```python
from build123d import *

# Parameters (mm, degrees)
F0_R          = 3
F0_R_2        = 2.5
F1_DEPTH      = 300
F2_R          = 2
F3_R          = 7
F5_DEPTH      = 30
F5_DEPTH_BACK = 30


# Not quite as in the source:
# - a feature names something its author has since deleted; it is built from what else it names


with BuildPart() as f1:
    # F0 (on Top) → F1 (new body)
    with BuildSketch(Plane.XY):
        with BuildLine():
            Line((18.15, -30), (30, -30))
            Line((30, -30), (30, -18.15))
            Line((30, -18.15), (27.5, -18.15))
            Line((27.5, -18.15), (27.5, -20.15))
            Line((27.5, -20.15), (21.5477069044, -20.15))
            ThreePointArc((21.5477069044, -20.15), (19.5, -15), (21.5477069044, -9.85))
            Line((21.5477069044, -9.85), (27.5, -9.85))
            Line((27.5, -9.85), (27.5, -11.85))
            Line((27.5, -11.85), (30, -11.85))
            Line((30, -11.85), (30, 11.85))
            Line((30, 11.85), (27.5, 11.85))
            Line((27.5, 11.85), (27.5, 9.85))
            Line((27.5, 9.85), (21.5477069044, 9.85))
            ThreePointArc((21.5477069044, 9.85), (19.5, 15), (21.5477069044, 20.15))
            Line((21.5477069044, 20.15), (27.5, 20.15))
            Line((27.5, 20.15), (27.5, 18.15))
            Line((27.5, 18.15), (30, 18.15))
            Line((30, 18.15), (30, 30))
            Line((30, 30), (18.15, 30))
            Line((18.15, 30), (18.15, 27.5))
            Line((18.15, 27.5), (20.15, 27.5))
            Line((20.15, 27.5), (20.15, 21.5477069044))
            ThreePointArc((20.15, 21.5477069044), (15, 19.5), (9.85, 21.5477069044))
            Line((9.85, 21.5477069044), (9.85, 27.5))
            Line((9.85, 27.5), (11.85, 27.5))
            Line((11.85, 27.5), (11.85, 30))
            Line((11.85, 30), (-11.85, 30))
            Line((-11.85, 30), (-11.85, 27.5))
            Line((-11.85, 27.5), (-9.85, 27.5))
            Line((-9.85, 27.5), (-9.85, 21.5477069044))
            ThreePointArc((-9.85, 21.5477069044), (-15, 19.5), (-20.15, 21.5477069044))
            Line((-20.15, 21.5477069044), (-20.15, 27.5))
            Line((-20.15, 27.5), (-18.15, 27.5))
            Line((-18.15, 27.5), (-18.15, 30))
            Line((-18.15, 30), (-30, 30))
            Line((-30, 30), (-30, 18.15))
            Line((-30, 18.15), (-27.5, 18.15))
            Line((-27.5, 18.15), (-27.5, 20.15))
            Line((-27.5, 20.15), (-21.5477069044, 20.15))
            ThreePointArc((-21.5477069044, 20.15), (-19.5, 15), (-21.5477069044, 9.85))
            Line((-21.5477069044, 9.85), (-27.5, 9.85))
            Line((-27.5, 9.85), (-27.5, 11.85))
            Line((-27.5, 11.85), (-30, 11.85))
            Line((-30, 11.85), (-30, -11.85))
            Line((-30, -11.85), (-27.5, -11.85))
            Line((-27.5, -11.85), (-27.5, -9.85))
            Line((-27.5, -9.85), (-21.5477069044, -9.85))
            ThreePointArc((-21.5477069044, -9.85), (-19.5, -15), (-21.5477069044, -20.15))
            Line((-21.5477069044, -20.15), (-27.5, -20.15))
            Line((-27.5, -20.15), (-27.5, -18.15))
            Line((-27.5, -18.15), (-30, -18.15))
            Line((-30, -18.15), (-30, -30))
            Line((-30, -30), (-18.15, -30))
            Line((-18.15, -30), (-18.15, -27.5))
            Line((-18.15, -27.5), (-20.15, -27.5))
            Line((-20.15, -27.5), (-20.15, -21.5477069044))
            ThreePointArc((-20.15, -21.5477069044), (-15, -19.5), (-9.85, -21.5477069044))
            Line((-9.85, -21.5477069044), (-9.85, -27.5))
            Line((-9.85, -27.5), (-11.85, -27.5))
            Line((-11.85, -27.5), (-11.85, -30))
            Line((-11.85, -30), (11.85, -30))
            Line((11.85, -30), (11.85, -27.5))
            Line((11.85, -27.5), (9.85, -27.5))
            Line((9.85, -27.5), (9.85, -21.5477069044))
            ThreePointArc((9.85, -21.5477069044), (15, -19.5), (20.15, -21.5477069044))
            Line((20.15, -21.5477069044), (20.15, -27.5))
            Line((20.15, -27.5), (18.15, -27.5))
            Line((18.15, -27.5), (18.15, -30))
        make_face()
        with Locations((-25, -25)):
            Circle(F0_R, mode=Mode.SUBTRACT)
        with Locations((-15, -15)):
            Circle(F0_R_2, mode=Mode.SUBTRACT)
        with Locations((25, -25)):
            Circle(F0_R, mode=Mode.SUBTRACT)
        with Locations((15, -15)):
            Circle(F0_R_2, mode=Mode.SUBTRACT)
        with Locations((-25, 25)):
            Circle(F0_R, mode=Mode.SUBTRACT)
        with Locations((-15, 15)):
            Circle(F0_R_2, mode=Mode.SUBTRACT)
        Polygon((-7, 22), (-7, 27.5), (0, 27.5), (7, 27.5), (7, 22), (10, 16), (10, 10), (16, 10), (22, 7), (27.5, 7), (27.5, 0), (27.5, -7), (22, -7), (16, -10), (10, -10), (10, -16), (7, -22), (7, -27.5), (0, -27.5), (-7, -27.5), (-7, -22), (-10, -16), (-10, -10), (-16, -10), (-22, -7), (-27.5, -7), (-27.5, 0), (-27.5, 7), (-22, 7), (-16, 10), (-10, 10), (-10, 16), align=None, mode=Mode.SUBTRACT)
        with Locations((15, 15)):
            Circle(F0_R_2, mode=Mode.SUBTRACT)
        with Locations((25, 25)):
            Circle(F0_R, mode=Mode.SUBTRACT)
    extrude(amount=F1_DEPTH)

    # F2
    f2_edges = [f1.edges().sort_by_distance(p)[0] for p in [
        (-7, 27.5, 150),
        (7, 27.5, 150),
    ]]
    fillet(f2_edges, radius=F2_R)

    # F3
    f3_edges = [f1.edges().sort_by_distance(p)[0] for p in [
        (-10, 16, 150),
        (10, 16, 150),
    ]]
    fillet(f3_edges, radius=F3_R)

    # F4 (on Right) → F5 (cut, two sides)
    with BuildSketch(Plane.YZ) as f5_sk:
        Polygon((-20.5082305996, 553.922022371), (-199.5184071674, 518.3146843648), (-149.0101765678, 264.3926619939), (30, 300), align=None)
    extrude(amount=F5_DEPTH, mode=Mode.SUBTRACT)
    extrude(f5_sk.sketch, amount=-F5_DEPTH_BACK, mode=Mode.SUBTRACT)


solid = f1.part
```
Check sheet for the modelled part. Datum: model origin and axes. Units: mm. Coordinates: 2 decimals unless noted, no trailing zeros. Loops run counter-clockwise (first coordinate to the right, second up) from the corner with the lowest first, then second, coordinate; pieces in that order, holes last. Notation, with made-up numbers: M 11.25,-30 L 59.25,-30 A20 cw 59.25,-11 Z; hole C 1,71.5 d2. An arc over 180 degrees is marked long. Answer as a JSON object with one key per item and string values.
1. Sectioned sample at B-B on y = -1. Record the cut outline in (x, z), and give its area (3 significant figures).
Outcome:
{"outline": "M -30,0 L -27.5,0 L -27.5,293.83 L -30,293.83 Z; M 27.5,0 L 30,0 L 30,293.83 L 27.5,293.83 Z", "area": "1,470 mm²"}
2. Sectioned sample at D-D on z = 121.5. Count the separate pieces of the cut face and the enclosed holes in it, and give its area (3 significant figures).
Outcome:
{"separate pieces": "1", "enclosed holes": "9", "area": "1,080 mm²"}
3. Sectioned sample at C-C on x = -25. Record the cut outline in (y, z).
Outcome:
{"outline": "M -30,0 L -28,0 L -28,288.46 L -30,288.07 Z; M -22,0 L -20.15,0 L -20.15,290.02 L -22,289.66 Z; M -9.85,0 L -7,0 L -7,292.64 L -9.85,292.07 Z; M 7,0 L 9.85,0 L 9.85,295.99 L 7,295.43 Z; M 20.15,0 L 22,0 L 22,298.41 L 20.15,298.04 Z; M 28,0 L 30,0 L 30,300 L 28,299.6 Z"}
4. Depth check by flat-ended pin: P1, Ø8, axis at x = -10.5, y = -3, coming from the -Z side; P2, Ø2, axis at x = -15, z = 262.5, coming from the +Y side. Enter the tip coordinate at first touch or a pass-through.
Outcome:
{"P1": "through", "P2": "y = 19.57"}
5. Release check for a two-part mould opening along Y. For faces 1 (the flat face through (-24, 30, 148)), 2 (the flat face through (-19, -8.5, 144.3)), 3 (the flat face through (30, 0, 146)) record: pulls with the +Y half, pulls with the -Y half, needs draft (parallel to the pull), parting line crosses it, or undercut.
Outcome:
{"face 1": "pulls with the +Y half", "face 2": "undercut", "face 3": "needs draft"}
6. Sectioned sample at A-A on x = -1.5. Record the cut outline in (y, z).
Outcome:
{"outline": "M -30,0 L -27.5,0 L -27.5,288.56 L -30,288.07 Z; M 27.5,0 L 30,0 L 30,300 L 27.5,299.5 Z"}
7. Scan lines: L1, parallel to X at y = 15, z = 190.5; L2, parallel to X at y = 15.5, z = 15; L3, parallel to Y at x = -15, z = 126. Record each from-to range of solid material in increasing order. Write a range as from..to.
Outcome:
{"L1": "-19.5..-17.5, -12.5..-9.97, 9.97..12.5, 17.5..19.5", "L2": "-19.52..-17.45, -12.55..-9.9, 9.9..12.55, 17.45..19.52", "L3": "-19.5..-17.5, -12.5..-10, 10..12.5, 17.5..19.5"}
